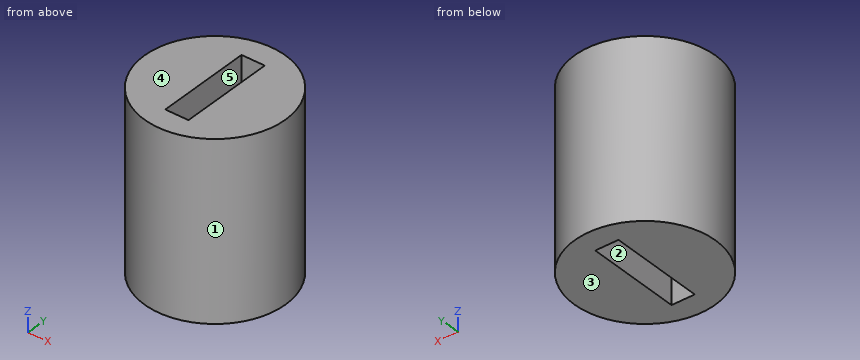
Autodesk Inventor part; units mm, degrees
ref_plane "YZ Plane" through (0, 0, 0) normal (1, 0, 0) x (0, 1, 0)
ref_plane "XZ Plane" through (0, 0, 0) normal (0, 1, 0) x (-1, 0, 0)
ref_plane "XY Plane" through (0, 0, 0) normal (0, 0, 1) x (1, 0, 0)
sketch "Эскиз1" plane through (0, 0, 0) normal (0, 0, 1) x (1, 0, 0)
  circle A0 centre (-31.2403, 27.0306) radius 4
  line L0 (-31.9005, 24.3212) -> (-30.5802, 24.3212)
  line L1 (-30.5802, 24.3212) -> (-30.5802, 29.74)
  line L2 (-30.5802, 29.74) -> (-31.9005, 29.74)
  line L3 (-31.9005, 29.74) -> (-31.9005, 24.3212)
  line L4 (-31.9005, 24.3212) -> (-30.5802, 29.74) construction
  line L5 (-30.5802, 24.3212) -> (-31.9005, 29.74) construction
  point P0 (0, 0)
  dimension "d0" = 8
extrude "Выдавливание1" add sketch "Эскиз1" along normal blind 10
ref_plane "РабПлоскость1" through (-63.6305, 53.4641, -0.3717) normal (0, 0, 1) x (1, 0, 0)
sketch "Эскиз2" plane through (-63.6305, 53.4641, -0.3717) normal (0, 0, 1) x (1, 0, 0)
  circle A0 centre (0, 0) radius 42.5 construction
  point P0 (63.6305, -53.4641)
  dimension "d3" = 85
properties part number "Clemma_CPY"
For this review, take the finished solid that the model builds, in its own axes (mm). Face numbers are marked on the shaded views. A direction names the side the tool comes from. Give positions to 0.01 mm unless a question says otherwise; leave off trailing zeros. Loops run counter-clockwise (first coordinate to the right, second up) from the corner with the lowest first, then second, coordinate; pieces in that order, holes last. Notation, with made-up numbers: M -36,25 L 8,25 A20 ccw 8,46 Z; hole C 32,-5.75 d7. An arc over 180 degrees is marked long. One line per item, written item: value. Start each with the question number.
Q1. Machinability: for the marked faces 4 and 5, which of the approach directions +Z, -Z, +X, -X, +Y, -Y give a long, thin tool a straight path to every point of the face, cutting with its end or side? Answer none if there is none.
Q2. Add section D-D (y = 30.25). Give the boundary of the cut face in (x, z).
Q3. Add section A-A (y = 26.25). Give the boundary of the cut face in (x, z).
Q4. For L1, parallel to Y at x = -31.5, z = 5.25; L2, parallel to X at y = 27, z = 7; L3, parallel to X at y = 29, z = 6.5, list the stretches that pass through material, from the lowest coordinate up.
Q5. Add section B-B (x = -31.5). Give the boundary of the cut face in (y, z), and give its area (3 significant figures).
Q6. Add section C-C (z = 2.75). Give the boundary of the cut face in (x, y), and give its area (3 significant figures).
Q7. Draft analysis for pull direction Y (two halves, no side actions). For the marked faces 1, 2 and 3, state which applies: released by +Y, released by -Y, zero draft, split by the parting line, or undercut.
Q8. Clearance check with flat-ended pins moving along their axes: pin 1 Ø2.5 at (y, z) = (26, 4.5) entering from -X; pin 2 Ø3 at (x, z) = (-33.5, 6.5) entering from +Y; pin 3 Ø1 at (x, z) = (-30.5, 3.5) entering from -Y. State where each tip first meets the part, or that it passes through.
Reply:
1. face 4: +Z, +X, -X, +Y, -Y
1. face 5: +Z, -Z
2. outline: M -33.61,0 L -28.87,0 L -28.87,10 L -33.61,10 Z
3. outline: M -35.16,0 L -31.9,0 L -31.9,10 L -35.16,10 Z; M -30.58,0 L -27.32,0 L -27.32,10 L -30.58,10 Z
4. L1: 23.04 to 24.32, 29.74 to 31.02
4. L2: -35.24 to -31.9, -30.58 to -27.24
4. L3: -34.72 to -31.9, -30.58 to -27.76
5. outline: M 23.04,0 L 24.32,0 L 24.32,10 L 23.04,10 Z; M 29.74,0 L 31.02,0 L 31.02,10 L 29.74,10 Z
5. area: 25.6 mm²
6. outline: C -31.24,27.03 d8; hole M -31.9,24.32 L -30.58,24.32 L -30.58,29.74 L -31.9,29.74 Z
6. area: 43.1 mm²
7. face 1: split by the parting line
7. face 2: undercut
7. face 3: zero draft
8. pin 1: x = -35.24
8. pin 2: y = 30.96
8. pin 3: y = 23.04
